The model under review builds one solid part; all positions refer to its coordinate system, in mm. Face numbers are marked on the shaded views. Round coordinates to 2 decimals unless told otherwise and drop trailing zeros. Order: outer loops, then holes, each group sorted by start corner. A loop starts at its lowest first (then second) coordinate and runs counter-clockwise, first axis right, second up. Notation, with made-up numbers: M 68,0 L 119,0 A33 ccw 119,32 Z; hole C 62.5,41 d6. An arc over 180 degrees is marked long. Answer as a JSON object with one key per item and string values. Group by question number.
1) Insertion check: pin 1 Ø1.5 at (x, z) = (14.5, 8) entering from -Y; pin 2 Ø2 at (x, z) = (15.5, 3.5) entering from +Y. Each pin has a flat end and moves straight along its axis. Give the tip position at first contact, or say it passes through.
2) Consider section D-D, the plane y = 5. Write out the cut boundary in (x, z), then the cut area to 3 significant figures.
3) Consider section B-B, the plane x = 14.5. Write out the cut boundary in (y, z), then the cut area to 3 significant figures.
4) To check wall thickness, follow line 1 (Y direction, x = 13.25, z = 2.75); line 2 (X direction, y = -2.5, z = 8.75); line 3 (X direction, y = -1.75, z = 6.75). State the ranges of each line that lie inside material, in increasing order.
5) The part is to be moulded in two halves that separate along X. For the marked faces 1, 2 and 3, say which applies: +X half, -X half, draft (parallel to the pull), parting line (faces both ways), or undercut.
6) Consider section C-C, the plane y = 2.5. Write out the cut boundary in (x, z), then the cut area to 3 significant figures.
```python
from build123d import *

# Parameters (mm, degrees)
F0_R        = 3.5
F1_DEPTH    = 10
F2_T1_DEPTH = 18.5839507528
F2_T3_DEPTH = 18.5839507528


# Not quite as in the source:
# - a fillet or chamfer that OpenCascade refuses, or shapes differently, is made with other operations: its cross-section is extruded or revolved along the edge and cut away or added


with BuildPart() as f1:
    # F0 (on Top) → F1 (new body)
    with BuildSketch(Plane.XY):
        with BuildLine():
            Line((17.4284250579, 4.5), (18.459414942, 4.5))
            ThreePointArc((18.459414942, 4.5), (18.1842599773, 5.507512059), (17.8541597949, 6.4983827232))
            Line((17.8541597949, 6.4983827232), (16.9144671741, 6.1563625799))
            ThreePointArc((16.9144671741, 6.1563625799), (17.191406166, 5.3343747558), (17.4284250579, 4.5))
        make_face()
        with BuildLine():
            ThreePointArc((17.8541597949, -6.4983827232), (18.1842599773, -5.507512059), (18.459414942, -4.5))
            Line((18.459414942, -4.5), (17.4284250579, -4.5))
            ThreePointArc((17.4284250579, -4.5), (17.191406166, -5.3343747558), (16.9144671741, -6.1563625799))
            Line((16.9144671741, -6.1563625799), (17.8541597949, -6.4983827232))
        make_face()
        with BuildLine():
            ThreePointArc((18.459414942, -4.5), (18.8643696409, -2.2661769682), (19, 0))
            ThreePointArc((19, 0), (18.8643696409, 2.2661769682), (18.459414942, 4.5))
            Line((18.459414942, 4.5), (17.4284250579, 4.5))
            ThreePointArc((17.4284250579, 4.5), (17.8565345328, 2.2680772647), (18, 0))
            ThreePointArc((18, 0), (17.8565345328, -2.2680772647), (17.4284250579, -4.5))
            Line((17.4284250579, -4.5), (18.459414942, -4.5))
        make_face()
        with BuildLine():
            ThreePointArc((18, 0), (17.8565345328, 2.2680772647), (17.4284250579, 4.5))
            Line((17.4284250579, 4.5), (13.4188298839, 4.5))
            ThreePointArc((13.4188298839, 4.5), (16.6008103993, 3.1819805153), (17.9188298839, 0))
            ThreePointArc((17.9188298839, 0), (16.6008103993, -3.1819805153), (13.4188298839, -4.5))
            Line((13.4188298839, -4.5), (17.4284250579, -4.5))
            ThreePointArc((17.4284250579, -4.5), (17.8565345328, -2.2680772647), (18, 0))
        make_face()
        with BuildLine():
            ThreePointArc((17.9188298839, 0), (16.6008103993, 3.1819805153), (13.4188298839, 4.5))
            ThreePointArc((13.4188298839, 4.5), (8.9188298839, 0), (13.4188298839, -4.5))
            ThreePointArc((13.4188298839, -4.5), (16.6008103993, -3.1819805153), (17.9188298839, 0))
        make_face()
        with Locations((13.4188298839, 0)):
            Circle(F0_R, mode=Mode.SUBTRACT)
    extrude(amount=F1_DEPTH)

    # F2: fillet of radius 2.25 on 2 edges, made by hand

    # F2_s2 → F2_t1 (cut)
    with BuildSketch(Plane.XY.offset(-4.2919753764)):
        with BuildLine():
            ThreePointArc((17.8541597949, 6.4983827232), (17.4032553622, 5.5588577913), (17.4240420287, 4.5169413745))
            ThreePointArc((17.4240420287, 4.5169413745), (17.1888111585, 5.342730665), (16.9144671741, 6.1563625799))
            Line((16.9144671741, 6.1563625799), (17.8541597949, 6.4983827232))
        make_face()
    extrude(amount=F2_T1_DEPTH, mode=Mode.SUBTRACT)

    # F2_s4 → F2_t3 (cut)
    with BuildSketch(Plane.XY.offset(-4.2919753764)):
        with BuildLine():
            ThreePointArc((17.8541597949, -6.4983827232), (17.4032553622, -5.5588577913), (17.4240420287, -4.5169413745))
            ThreePointArc((17.4240420287, -4.5169413745), (17.1888111585, -5.342730665), (16.9144671741, -6.1563625799))
            Line((16.9144671741, -6.1563625799), (17.8541597949, -6.4983827232))
        make_face()
    extrude(amount=F2_T3_DEPTH, mode=Mode.SUBTRACT)


solid = f1.part
```
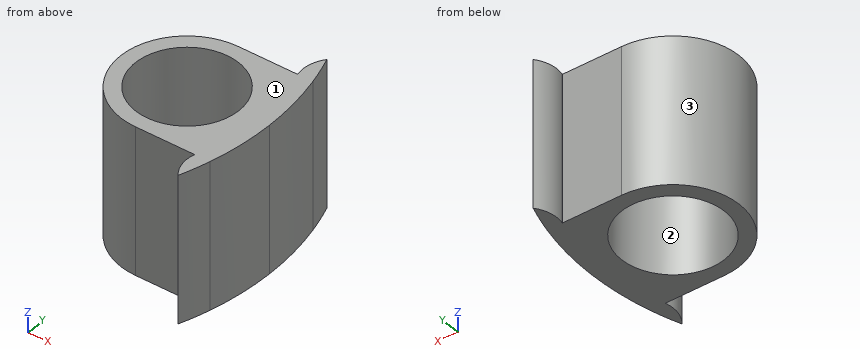
Results list:
{
 "1": {"pin 1": "y = -4.5", "pin 2": "y = 4.5"},
 "2": {"outline": "M 17.35,0 L 18.33,0 L 18.33,10 L 17.35,10 Z", "area": "9.77 mm^2"},
 "3": {"outline": "M -4.5,0 L -3.33,0 L -3.33,10 L -4.5,10 Z; M 3.33,0 L 4.5,0 L 4.5,10 L 3.33,10 Z", "area": "23.4 mm^2"},
 "4": {"line 1": "-4.5 to -3.5, 3.5 to 4.5", "line 2": "9.68 to 10.97, 15.87 to 18.83", "line 3": "9.27 to 10.39, 16.45 to 18.92"},
 "5": {"face 1": "draft", "face 2": "undercut", "face 3": "-X half"},
 "6": {"outline": "M 9.68,0 L 10.97,0 L 10.97,10 L 9.68,10 Z; M 15.87,0 L 18.83,0 L 18.83,10 L 15.87,10 Z", "area": "42.6 mm^2"}
}
